Here's the drawing with two shaded views (mm, measured from the low corner). I have some questions. Coordinates: 2 decimals unless noted, no trailing zeros. Loops run counter-clockwise (first coordinate to the right, second up) from the corner with the lowest first, then second, coordinate; pieces in that order, holes last. Notation, with made-up numbers: (20.25, 83.5) - (67.25, 83.5) arc R33 cw to (67.25, 113.5) - close; hole circle Ø10 at (0.25, -34.5). An arc over 180 degrees is marked (long way). One line per item, written item: value. Start each with the question number.
(1) If we section it at D-D on x = 35: Write out the boundary of the cut face in (y, z).
(2) I'm going to push flat-ended pins straight in: P1, Ø1, axis at x = 29, z = 1, coming from the -Y side; P2, Ø1, axis at y = 103.5, z = 1, coming from the -X side; P3, Ø1.5, axis at x = 1.5, z = 1, coming from the +Y side. Where does each tip first touch, or does it pass through?
(3) If we section it at B-B on z = 2.05: Count the separate pieces of the cut face and the enclosed holes in it, then the cut area to 3 significant figures.
(4) If we section it at C-C on y = 103: Write out the boundary of the cut face in (x, z), then the cut area to 3 significant figures.
(5) If I drill on line 1 along X through (y, z) = (67, 2.1); line 2 along X through (y, z) = (79, 2.1); line 3 along Y through (x, z) = (59, 2.2), over which ranges is the centre line in solid material (lowest first)? Write a range as from..to.
(6) If we section it at A-A on y = 70: Write out the boundary of the cut face in (x, z), then the cut area to 3 significant figures.
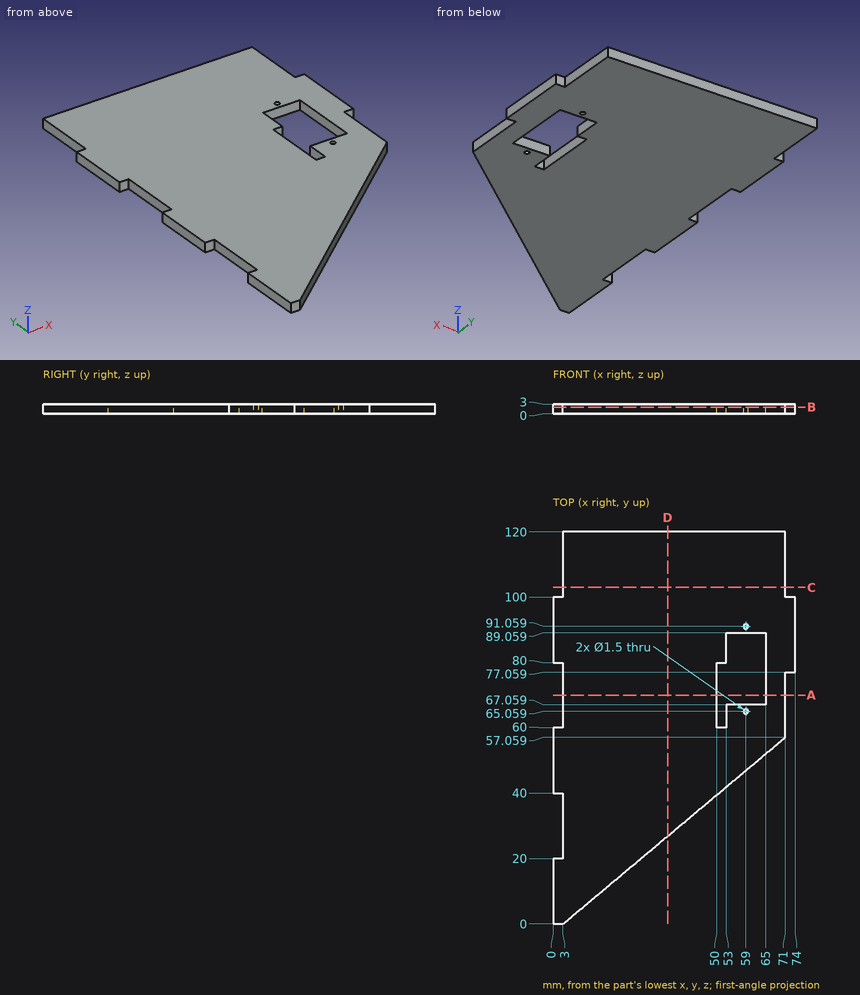
Values:
1. outline: (26.85, 0) - (120, 0) - (120, 3) - (26.85, 3) - close
2. P1: stops at y = 21.4
2. P2: stops at x = 3
2. P3: stops at y = 100
3. separate pieces: 1
3. enclosed holes: 3
3. area: 6,140 mm2
4. outline: (3, 0) - (71, 0) - (71, 3) - (3, 3) - close
4. area: 204 mm2
5. line 1: x = 3..50, 53..71
5. line 2: x = 3..50, 65..74
5. line 3: y = 46.99..64.31, 65.81..67.06, 89.06..90.31, 91.81..120
6. outline: (3, 0) - (50, 0) - (50, 3) - (3, 3) - close; (65, 0) - (71, 0) - (71, 3) - (65, 3) - close
6. area: 159 mm2
